Can you work these out from the drawing? Everything is in mm from the part's minimum corner. A direction names the side the tool comes from. Give positions to 0.01 mm unless a question says otherwise; leave off trailing zeros. Loops run counter-clockwise (first coordinate to the right, second up) from the corner with the lowest first, then second, coordinate; pieces in that order, holes last. Notation, with made-up numbers: (73, 54) - (118, 54) arc R12 cw to (118, 59) - close; hole circle Ø6 at (46.5, 24). An arc over 180 degrees is marked (long way). Answer in a Markdown table with one row per item.
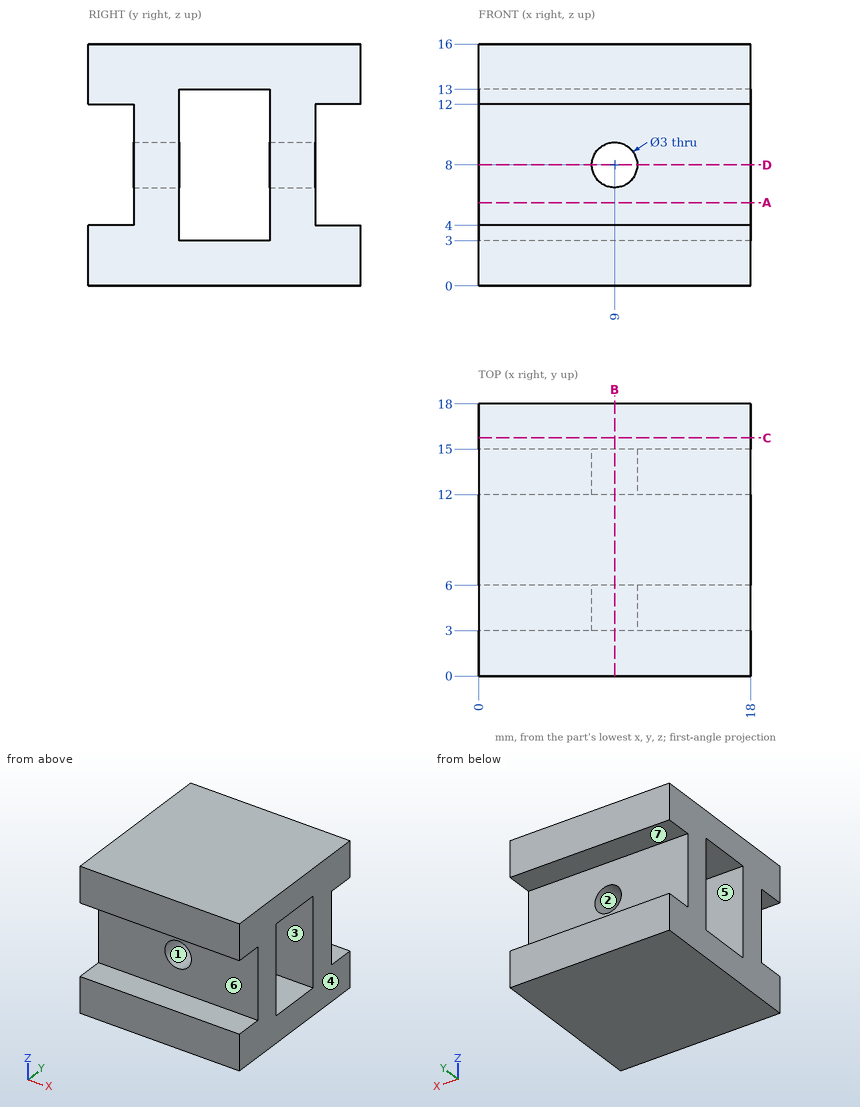
Q1. Imagine slicing it at D-D, the plane z = 8. Write out the boundary of the cut face in (x, y), and give its area (3 significant figures).
Checked values:
| item | result |
|---|---|
| outline | (0, 3) - (7.5, 3) - (7.5, 6) - (0, 6) - close; (0, 12) - (7.5, 12) - (7.5, 15) - (0, 15) - close; (10.5, 3) - (18, 3) - (18, 6) - (10.5, 6) - close; (10.5, 12) - (18, 12) - (18, 15) - (10.5, 15) - close |
| area | 90.0 mm² |
Q2. Imagine slicing it at C-C, the plane y = 15.75. Write out the boundary of the cut face in (x, z), and give its area (3 significant figures).
Checked values:
| item | result |
|---|---|
| outline | (0, 0) - (18, 0) - (18, 4) - (0, 4) - close; (0, 12) - (18, 12) - (18, 16) - (0, 16) - close |
| area | 144 mm² |
Q3. If I drill on line 1 (Z direction, x = 2, y = 16.5); line 2 (Z direction, x = 9, y = 4.2); line 3 (X direction, y = 4.4, z = 8), over which ranges is the centre line in solid material (lowest first)? Write a range as [from, to].
Checked values:
| item | result |
|---|---|
| line 1 | z = [0, 4], [12, 16] |
| line 2 | z = [0, 6.5], [9.5, 16] |
| line 3 | x = [0, 7.5], [10.5, 18] |
Q4. For pin 1 (2.5 mm diameter, centred on x = 7, z = 9.5, fed in from +Y); pin 2 (2.5 mm diameter, centred on x = 12.5, z = 7, fed in from -Y), each with a flat end and sliding along its axis, tell me the tip position at first contact or that it passes through.
Checked values:
| item | result |
|---|---|
| pin 1 | stops at y = 15 |
| pin 2 | stops at y = 3 |
Q5. On a 3-axis mill with a long thin cutter (end or side, diameter ignored), from which of +Z, -Z, +X, -X, +Y, -Y can I reach the whole of each face in a straight line? I mean the marked faces 5, 6 and 7. Say none if no direction works.
Checked values:
| item | result |
|---|---|
| face 5 | +X, -X |
| face 6 | +X, -X, -Y |
| face 7 | +X, -X, +Y |
Q6. Imagine slicing it at A-A, the plane z = 5.5. Write out the boundary of the cut face in (x, y).
Checked values:
| item | result |
|---|---|
| outline | (0, 3) - (18, 3) - (18, 6) - (0, 6) - close; (0, 12) - (18, 12) - (18, 15) - (0, 15) - close |
Q7. If we mould it in two halves opening along X, with no side actions, what happens to the marked faces 1, 2, 3 and 4? For each: released by +X, released by -X, zero draft, split by the parting line, or undercut.
Checked values:
| item | result |
|---|---|
| face 1 | undercut |
| face 2 | undercut |
| face 3 | zero draft |
| face 4 | released by +X |
Q8. Imagine slicing it at B-B, the plane x = 9. Write out the boundary of the cut face in (y, z), and give its area (3 significant figures).
Checked values:
| item | result |
|---|---|
| outline | (0, 0) - (18, 0) - (18, 4) - (15, 4) - (15, 6.5) - (12, 6.5) - (12, 3) - (6, 3) - (6, 6.5) - (3, 6.5) - (3, 4) - (0, 4) - close; (0, 12) - (3, 12) - (3, 9.5) - (6, 9.5) - (6, 13) - (12, 13) - (12, 9.5) - (15, 9.5) - (15, 12) - (18, 12) - (18, 16) - (0, 16) - close |
| area | 162 mm² |
